from build123d import *

# Parameters (mm, degrees)
SKETCH1_R           = 1.7
BOSS_EXTRUDE3_DEPTH = 30
SKETCH3_W           = 15
SKETCH3_H           = 24
SKETCH3_H_2         = 20
CUT_EXTRUDE1_DEPTH  = 30


with BuildPart() as part:
    # Sketch1 → Boss-Extrude3 (new body)
    with BuildSketch(Plane(origin=(0, 0, 0), x_dir=(1, 0, 0), z_dir=(0, 1, 0))):
        with BuildLine():
            Line((-5.313882261, 48.296626618), (-9.168605584, 46.167598374))
            Line((-9.168605584, 46.167598374), (11.814117054, 11.491925283))
            Line((11.814117054, 11.491925283), (12.539193688, 10.293676573))
            ThreePointArc((12.539193688, 10.293676573), (18.482268259, 9.569826652), (19.671887971, 15.437441074))
            Line((19.671887971, 15.437441074), (1.001872335, 46.167598374))
            Line((1.001872335, 46.167598374), (0.516004793, 46.873367152))
            ThreePointArc((0.516004793, 46.873367152), (-2.104172047, 48.792406027), (-5.313882261, 48.296626618))
        make_face()
        with Locations(Location((15.902373856, 13.147283989, 0), (0, 0, 270))):
            Circle(SKETCH1_R, mode=Mode.SUBTRACT)
        with Locations(Location((-3.110568467, 44.670053358, 0), (0, 0, 270))):
            Circle(SKETCH1_R, mode=Mode.SUBTRACT)
    extrude(amount=BOSS_EXTRUDE3_DEPTH)

    # Sketch3 → Cut-Extrude1 (cut)
    with BuildSketch(Plane(origin=(13.737778319, 0, -8.312916994), x_dir=(0.5177090511258458, 0, 0.8555567417666561), z_dir=(-0.8555567417666561, 0, 0.5177090511258458))):
        with Locations((-36.745670137, 15)):
            Rectangle(SKETCH3_W, SKETCH3_H)
        with Locations((-6.104769326, 15)):
            Rectangle(SKETCH3_W, SKETCH3_H_2)
    extrude(amount=-CUT_EXTRUDE1_DEPTH, mode=Mode.SUBTRACT)


solid = part.part
Work out the finished part from the listing and answer in its coordinate system (mm). A direction names the side the tool comes from. Coordinates: 2 decimals unless noted, no trailing zeros. Order: outer loops, then holes, each group sorted by start corner. A loop starts at its lowest first (then second) coordinate and runs counter-clockwise, first axis right, second up. Notation, with made-up numbers: (49, 19) - (74, 19) arc R33 ccw to (74, 53) - close; hole circle Ø4 at (22, -22). An arc over 180 degrees is marked (long way). Put each result on its own line as item: value. Start each with the question number.
1) Find section A-A (y = 4). Give the vertices of the cut face in (x, z).
2) Find the intervals of material crossed by line 1 (Y direction, x = -4.75, z = -44); line 2 (Z direction, x = 16.5, y = 28); line 3 (Z direction, x = 9.5, y = 4), in increasing order. Write a range as from..to.
3) For faces 1 (the flat face through (14, 5, -16)), 2 (the flat face through (-2, 3, -42)), 3 (the flat face through (10.468, 14.79, -30.587)), determine the directions among +Z, -Z, +X, -X, +Y, -Y from which every point of the face is accessible in a straight line to the end or side of a thin tool.
4) Flat-ended cylindrical pins translate along their axes: pin 1 (1 mm diameter, centred on x = -0.5, y = 14, fed in from +Z); pin 2 (4 mm diameter, centred on y = 3.5, z = -35.5, fed in from -X); pin 3 (2 mm diameter, centred on x = -3.11, z = -44.67, fed in from +Y); pin 4 (8 mm diameter, centred on x = 13, y = 21, fed in from -Z). Find the tip coordinate at first contact, or state that the pin passes through.
5) Find section D-D (x = 9.5). Give the vertices of the cut face in (y, z), plus the area to 3 significant figures.
6) For a pull along Y with two mould halves and no side action, classify faces 4 (the flat face through (2.275, 14.832, -35.56)), 5 (the cylindrical face through (-3.04, 1.48, -46.37)), 6 (the flat face through (7, 0, -29)) as released by +Y, released by -Y, zero draft, split by the parting line, or undercut.
7) Find section B-B (x = -2). Give the vertices of the cut face in (y, z).
8) Find section C-C (z = -40). Give the vertices of the cut face in (x, y).
Results list:
1. outline: (-1.4, -33.33) - (6.06, -37.85) - (19.67, -15.44) arc R4.41 ccw to (12.54, -10.29) - close; hole circle Ø3.4 at (15.9, -13.15)
2. line 1: y = 0..3, 27..30
2. line 2: z = -20.66..-14.74, -11.56..-8.78
2. line 3: z = -32.18..-15.32
3. face 1: +Z, +X
3. face 2: -Z, -X
3. face 3: -Z, +X, +Y, -Y
4. pin 1: stops at z = -31.02
4. pin 2: stops at x = -3.89
4. pin 3: passes through
4. pin 4: stops at z = -33
5. outline: (0, -32.18) - (30, -32.18) - (30, -15.32) - (25, -15.32) - (25, -21.65) - (5, -21.65) - (5, -15.32) - (0, -15.32) - close
5. area: 379 mm^2
6. face 4: undercut
6. face 5: zero draft
6. face 6: released by -Y
7. outline: (0, -48.77) - (3, -48.77) - (3, -45.96) - (0, -45.96) - close; (0, -43.38) - (3, -43.38) - (3, -34.32) - (0, -34.32) - close; (27, -48.77) - (30, -48.77) - (30, -45.96) - (27, -45.96) - close; (27, -43.38) - (30, -43.38) - (30, -34.32) - (27, -34.32) - close
8. outline: (-5.44, 0) - (4.75, 0) - (4.75, 3) - (-5.44, 3) - close; (-5.44, 27) - (4.75, 27) - (4.75, 30) - (-5.44, 30) - close
